```python
from build123d import *

# Parameters (mm, degrees)
F0_W     = 50
F0_H     = 100
F1_DEPTH = 800
F3_DEPTH = 50.001


with BuildPart() as f1:
    # F0 (on Front) → F1 (new body)
    with BuildSketch(Plane.XZ):
        with Locations((25, 50)):
            Rectangle(F0_W, F0_H)
    extrude(amount=F1_DEPTH)

    # F2 (on face) → F3 (cut, through all)
    with BuildSketch(Plane.YZ.offset(50)):
        with BuildLine():
            Line((-715, 100), (-755, 100))
            ThreePointArc((-755, 100), (-735, 80), (-715, 100))
        make_face()
        with BuildLine():
            Line((-65, 100), (-105, 100))
            ThreePointArc((-105, 100), (-85, 80), (-65, 100))
        make_face()
    extrude(amount=-F3_DEPTH, mode=Mode.SUBTRACT)


solid = f1.part
```
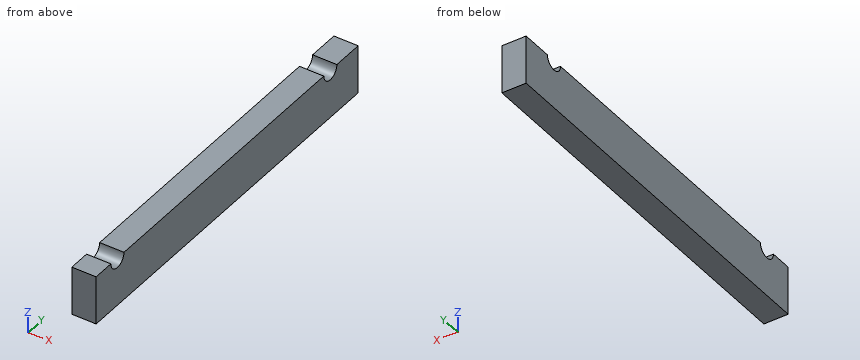
Check sheet for the modelled part. Datum: model origin and axes. Units: mm. Round coordinates to 2 decimals unless told otherwise and drop trailing zeros. Loops run counter-clockwise (first coordinate to the right, second up) from the corner with the lowest first, then second, coordinate; pieces in that order, holes last. Notation, with made-up numbers: (-1.5, 11) - (49.5, 11) arc R32 ccw to (49.5, 40) - close; hole circle Ø1 at (53.5, -32). An arc over 180 degrees is marked (long way). Answer as a JSON object with one key per item and string values. Group by question number.
Q1. Sectioned sample at B-B, the plane y = -85. Enter the section's corners in (x, z), plus the area to 3 significant figures.
Q2. Scan line: line 1 along Y through (x, z) = (17, 94). Record every from-to range of solid material in increasing order. Write a range as [from, to].
Q3. Sectioned sample at A-A, the plane x = 21.5. Enter the section's corners in (y, z), plus the area to 3 significant figures.
Solution:
{
 "1": {"outline": "(0, 0) - (50, 0) - (50, 80) - (0, 80) - close", "area": "4,000 mm²"},
 "2": {"line 1": "y = [-800, -754.08], [-715.92, -104.08], [-65.92, 0]"},
 "3": {"outline": "(-800, 0) - (0, 0) - (0, 100) - (-65, 100) arc R20 cw to (-105, 100) - (-715, 100) arc R20 cw to (-755, 100) - (-800, 100) - close", "area": "78,700 mm²"}
}
